```python
from build123d import *

# Parameters (mm, degrees)
F0_R     = 17
F0_R_2   = 58
F1_DEPTH = 10


with BuildPart() as f1:
    # F0 (on Top) → F1 (new body)
    with BuildSketch(Plane.XY):
        with BuildLine():
            add(Edge.make_bspline(
                [(-25.6339077997, -554.9584652973), (-51.3281857013, -553.7520074813), (-93.6695279871, -547.7281922836), (-112.8758760553, -542.5469908858)],
                knots=[0, 0, 0, 0, 1, 1, 1, 1], degree=3))
            add(Edge.make_bspline(
                [(101.8517638204, -546.5538520712), (75.6875139287, -553.2760310818), (18.5277424792, -557.0443555931), (-25.6339077997, -554.9584652973)],
                knots=[0, 0, 0, 0, 1, 1, 1, 1], degree=3))
            add(Edge.make_bspline(
                [(196.2248278388, -479.4811160712), (171.822081153, -518.0226613149), (144.728786774, -537.2783267828), (101.8517638204, -546.5538520712)],
                knots=[0, 0, 0, 0, 1, 1, 1, 1], degree=3))
            add(Edge.make_bspline(
                [(215.5120574316, -395.3010671859), (217.1466194612, -422.7158916841), (209.2029400354, -457.3865119018), (196.2248278388, -479.4811160712)],
                knots=[0, 0, 0, 0, 1, 1, 1, 1], degree=3))
            add(Edge.make_bspline(
                [(192.3294851646, -312.5904306206), (210.6460825929, -360.2347591492), (213.5839387817, -370.7164733528), (215.5120574316, -395.3010671859)],
                knots=[0, 0, 0, 0, 1, 1, 1, 1], degree=3))
            add(Edge.make_bspline(
                [(169.7994317014, -220.6377759274), (170.8927200615, -250.1742175661), (174.6979485759, -265.704673421), (192.3294851646, -312.5904306206)],
                knots=[0, 0, 0, 0, 1, 1, 1, 1], degree=3))
            add(Edge.make_bspline(
                [(171.8513537255, -172.9866951147), (169.5959356869, -196.170976202), (169.2566540986, -204.0498641717), (169.7994317014, -220.6377759274)],
                knots=[0, 0, 0, 0, 1, 1, 1, 1], degree=3))
            add(Edge.make_bspline(
                [(156.5171346692, -69.2568868796), (174.5323214434, -93.697017447), (177.6080524724, -114.5030664178), (171.8513537255, -172.9866951147)],
                knots=[0, 0, 0, 0, 1, 1, 1, 1], degree=3))
            add(Edge.make_bspline(
                [(123.2144497533, -35.5076734554), (137.3923515164, -47.479706869), (149.9416092694, -60.1972288193), (156.5171346692, -69.2568868796)],
                knots=[0, 0, 0, 0, 1, 1, 1, 1], degree=3))
            add(Edge.make_bspline(
                [(65.3255478686, 58.7055848673), (71.3094857176, 18.2698117865), (84.0455293395, -2.4578782981), (123.2144497533, -35.5076734554)],
                knots=[0, 0, 0, 0, 1, 1, 1, 1], degree=3))
            Line((65.3255478686, 58.7055848673), (64.565721553, 64.4665316539))
            Line((64.565721553, 64.4665316539), (-52.3039117597, 64.4665316539))
            add(Edge.make_bspline(
                [(-53.2111279718, 58.9898998943), (-52.85822859, 60.9062352781), (-52.5589473666, 62.6516212459), (-52.3039117597, 64.4665316539)],
                knots=[0, 0, 0, 0, 0.1687767432, 0.1687767432, 0.1687767432, 0.1687767432], degree=3))
            add(Edge.make_bspline(
                [(-83.9275562826, -5.3117870477), (-68.5191745861, 10.9552480289), (-57.925205972, 33.1326502537), (-53.2111279718, 58.9898998943)],
                knots=[0, 0, 0, 0, 1, 1, 1, 1], degree=3))
            add(Edge.make_bspline(
                [(-116.1044629089, -32.9178178076), (-105.0576364154, -24.5577063166), (-89.4816840216, -11.1943914798), (-83.9275562826, -5.3117870477)],
                knots=[0, 0, 0, 0, 1, 1, 1, 1], degree=3))
            add(Edge.make_bspline(
                [(-151.7732536447, -67.2104688142), (-145.4823496584, -58.8826067666), (-127.2181132715, -41.3230190468), (-116.1044629089, -32.9178178076)],
                knots=[0, 0, 0, 0, 1, 1, 1, 1], degree=3))
            add(Edge.make_bspline(
                [(-167.8786038958, -100.9023919243), (-165.7922728196, -91.5504220926), (-158.2096647421, -75.6878301404), (-151.7732536447, -67.2104688142)],
                knots=[0, 0, 0, 0, 1, 1, 1, 1], degree=3))
            add(Edge.make_bspline(
                [(-171.0060882933, -126.3918295099), (-171.6524429426, -123.6316115462), (-170.0516423645, -110.5848282174), (-167.8786038958, -100.9023919243)],
                knots=[0, 0, 0, 0, 1, 1, 1, 1], degree=3))
            add(Edge.make_bspline(
                [(-169.5117163, -149.5662211718), (-170.0493651796, -138.0408590498), (-170.7218331806, -127.612381277), (-171.0060882933, -126.3918295099)],
                knots=[0, 0, 0, 0, 1, 1, 1, 1], degree=3))
            add(Edge.make_bspline(
                [(-167.471540599, -182.8861909723), (-168.0820735931, -176.0867543832), (-169.0001494598, -161.0927678386), (-169.5117163, -149.5662211718)],
                knots=[0, 0, 0, 0, 1, 1, 1, 1], degree=3))
            add(Edge.make_bspline(
                [(-169.8114988663, -236.5880074419), (-167.2539474938, -220.4051955184), (-166.2455341108, -197.26217001), (-167.471540599, -182.8861909723)],
                knots=[0, 0, 0, 0, 1, 1, 1, 1], degree=3))
            add(Edge.make_bspline(
                [(-191.3924597661, -298.1748905383), (-179.0718659588, -271.0675724162), (-172.1596309655, -251.3416179851), (-169.8114988663, -236.5880074419)],
                knots=[0, 0, 0, 0, 1, 1, 1, 1], degree=3))
            add(Edge.make_bspline(
                [(-211.7698147273, -349.4178452311), (-208.0178282467, -335.8281697152), (-203.8558661958, -325.3620944905), (-191.3924597661, -298.1748905383)],
                knots=[0, 0, 0, 0, 1, 1, 1, 1], degree=3))
            add(Edge.make_bspline(
                [(-211.9194493318, -449.6959373576), (-221.9116183428, -415.102756195), (-221.8712504731, -388.0341277686), (-211.7698147273, -349.4178452311)],
                knots=[0, 0, 0, 0, 1, 1, 1, 1], degree=3))
            add(Edge.make_bspline(
                [(-184.4620737021, -499.4476777279), (-195.4772493714, -486.0997058769), (-206.5682443762, -466.0032882637), (-211.9194493318, -449.6959373576)],
                knots=[0, 0, 0, 0, 1, 1, 1, 1], degree=3))
            add(Edge.make_bspline(
                [(-112.8758760553, -542.5469908858), (-142.243597994, -535.1274441055), (-168.6109492663, -519.252627116), (-184.4620737021, -499.4476777279)],
                knots=[0, 0, 0, 0, 1, 1, 1, 1], degree=3))
        make_face()
        with Locations((-1.1947170427, -404.1430069365)):
            Circle(F0_R, mode=Mode.SUBTRACT)
        with Locations((0.0564528571, -195.3839299387)):
            Circle(F0_R_2, mode=Mode.SUBTRACT)
    extrude(amount=F1_DEPTH)


solid = f1.part
```
The model under review builds one solid part; all positions refer to its coordinate system, in mm. Round coordinates to 2 decimals unless told otherwise and drop trailing zeros. Write item = value, one per line.
Item 1: Take a section at A-A on z = 2. State how many separate pieces and enclosed holes the cut face has, then the cut area to 3 significant figures.
Return value:
separate_pieces = 1
enclosed_holes = 2
area = 191,000 mm2
Item 2: Insertion check: P1, Ø1.5, axis at x = -120.5, z = 4.5, coming from the +Y side; P2, Ø6, axis at x = -37.5, z = 4.5, coming from the -Y side; P3, Ø1.5, axis at y = -418, z = 8, coming from the +X side; P4, Ø20.5, axis at x = -1.19, y = -404.14, coming from the +Z side. Each pin has a flat end and moves straight along its axis. Give the tip position at first contact, or say it passes through.
Return value:
P1 = -35.79
P2 = -554.41
P3 = 214.98
P4 = through
Item 3: The part is to be moulded in two halves that separate along X. For faces 1 (the flat face through (1, -311, 0)), 2 (the cylindrical face through (-7.494, -137.877, 4.93)), say which applies: released by +X, released by -X, zero draft, split by the parting line, or undercut.
Return value:
face_1 = zero draft
face_2 = undercut
Item 4: For line 1 (Y direction, x = 7.5, z = 2.5); line 2 (Y direction, x = 8, z = 1.5); line 3 (X direction, y = -182.5, z = 8.25), list the stretches that pass through material, from the lowest coordinate up. Write a range as [from, to].
Return value:
line_1 = [-555.49, -418.75], [-389.53, -252.9], [-137.86, 64.47]
line_2 = [-555.49, -418.44], [-389.84, -252.84], [-137.93, 64.47]
line_3 = [-167.51, -56.49], [56.61, 170.96]
